Part print with two shaded views. Sizes in mm from the minimum x, y, z corner. A direction names the side the tool comes from. Round coordinates to 2 decimals unless told otherwise and drop trailing zeros. Write each loop counter-clockwise with the first axis right and the second up, starting at its lowest first coordinate (ties: lowest second). Pieces come first, ordered by that corner, then holes. Notation, with made-up numbers: (11.5, 61) -> (44.5, 61) arc R23 ccw to (44.5, 80) -> close; hole circle Ø1 at (66.5, 80). An arc over 180 degrees is marked (long way). Return JSON: item names as keys, results as strings.
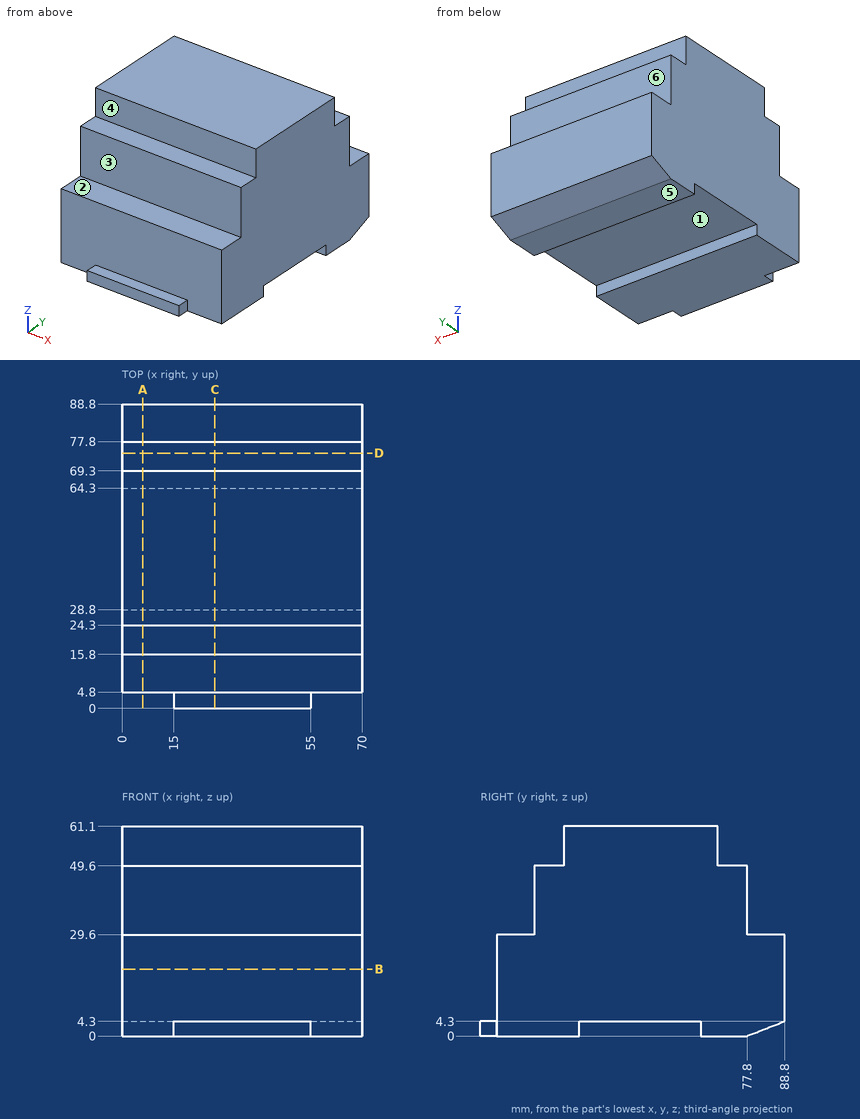
Q1. Pin check, flat tips, straight feed: pin 1 Ø12.5 at (x, z) = (18.5, 53.5) entering from +Y; pin 2 Ø9.5 at (x, y) = (24.5, 74.5) entering from +Z; pin 3 Ø1.4 at (x, y) = (35, 3.5) entering from +Z. Stop position of each tip, or through.
Verdict:
{"pin 1": "stops at y = 77.8", "pin 2": "stops at z = 49.6", "pin 3": "stops at z = 4.3"}
Q2. Wall check: L1, parallel to Y at x = 6, z = 50.5; L2, parallel to Y at x = 43, z = 14.5; L3, parallel to Z at x = 61.5, y = 40.5. Give the ranges that are in metal, low to high.
Verdict:
{"L1": "y = 24.3 to 69.3", "L2": "y = 4.8 to 88.8", "L3": "z = 4.3 to 61.1"}
Q3. Saw through at C-C on x = 27. List the corners of the cut face in (y, z).
Verdict:
{"outline": "(0, 0) -> (28.8, 0) -> (28.8, 4.3) -> (64.3, 4.3) -> (64.3, 0) -> (77.8, 0) -> (88.8, 4.3) -> (88.8, 29.6) -> (77.8, 29.6) -> (77.8, 49.6) -> (69.3, 49.6) -> (69.3, 61.1) -> (24.3, 61.1) -> (24.3, 49.6) -> (15.8, 49.6) -> (15.8, 29.6) -> (4.8, 29.6) -> (4.8, 4.3) -> (0, 4.3) -> close"}
Q4. Two-plate mould, pull along Y, no slides. Class the marked faces 1, 2 and 3: +Y half, -Y half, draft (parallel to the pull), parting line (faces both ways), or undercut.
Verdict:
{"face 1": "undercut", "face 2": "draft", "face 3": "-Y half"}
Q5. Saw through at A-A on x = 6. List the corners of the cut face in (y, z).
Verdict:
{"outline": "(4.8, 0) -> (28.8, 0) -> (28.8, 4.3) -> (64.3, 4.3) -> (64.3, 0) -> (77.8, 0) -> (88.8, 4.3) -> (88.8, 29.6) -> (77.8, 29.6) -> (77.8, 49.6) -> (69.3, 49.6) -> (69.3, 61.1) -> (24.3, 61.1) -> (24.3, 49.6) -> (15.8, 49.6) -> (15.8, 29.6) -> (4.8, 29.6) -> close"}
Q6. Saw through at B-B on z = 19.5. List the corners of the cut face in (x, y), then the cut area to 3 significant figures.
Verdict:
{"outline": "(0, 4.8) -> (70, 4.8) -> (70, 88.8) -> (0, 88.8) -> close", "area": "5,880 mm²"}
Q7. Saw through at D-D on y = 74.5. List the corners of the cut face in (x, z), then the cut area to 3 significant figures.
Verdict:
{"outline": "(0, 0) -> (70, 0) -> (70, 49.6) -> (0, 49.6) -> close", "area": "3,470 mm²"}
Q8. 3-axis set-ups, long thin cutter, end or side, ignore diameter. For the marked faces 4, 5 and 6: which of +Z, -Z, +X, -X, +Y, -Y reach the whole face in a straight line?
Verdict:
{"face 4": "+Z, +X, -X, -Y", "face 5": "-Z, +X, -X, +Y, -Y", "face 6": "+Z, +X, -X, +Y"}
